```python
from build123d import *

# Parameters (mm, degrees)
SKETCH1_R           = 13.5
BOSS_EXTRUDE1_DEPTH = 3.25
CUT_EXTRUDE1_DEPTH  = 4.25
FILLET1_R           = 0.57
CIRPATTERN3_COUNT   = 16


with BuildPart() as part:
    # Sketch1 → Boss-Extrude1 (new body, symmetric)
    with BuildSketch(Plane.XY):
        Circle(SKETCH1_R)
        with BuildLine():
            Line((1.4, 1), (2.1, 1))
            ThreePointArc((2.1, 1), (2.382842712, 0.882842712), (2.5, 0.6))
            Line((2.5, 0.6), (2.5, -0.6))
            ThreePointArc((2.5, -0.6), (2.382842712, -0.882842712), (2.1, -1))
            Line((2.1, -1), (1.4, -1))
            ThreePointArc((1.4, -1), (1.117157288, -1.117157288), (1, -1.4))
            Line((1, -1.4), (1, -2.1))
            ThreePointArc((1, -2.1), (0.882842712, -2.382842712), (0.6, -2.5))
            Line((0.6, -2.5), (-0.6, -2.5))
            ThreePointArc((-0.6, -2.5), (-0.882842712, -2.382842712), (-1, -2.1))
            Line((-1, -2.1), (-1, -1.4))
            ThreePointArc((-1, -1.4), (-1.117157288, -1.117157288), (-1.4, -1))
            Line((-1.4, -1), (-2.1, -1))
            ThreePointArc((-2.1, -1), (-2.382842712, -0.882842712), (-2.5, -0.6))
            Line((-2.5, -0.6), (-2.5, 0.6))
            ThreePointArc((-2.5, 0.6), (-2.382842712, 0.882842712), (-2.1, 1))
            Line((-2.1, 1), (-1.4, 1))
            ThreePointArc((-1.4, 1), (-1.117157288, 1.117157288), (-1, 1.4))
            Line((-1, 1.4), (-1, 2.1))
            ThreePointArc((-1, 2.1), (-0.882842712, 2.382842712), (-0.6, 2.5))
            Line((-0.6, 2.5), (0.6, 2.5))
            ThreePointArc((0.6, 2.5), (0.882842712, 2.382842712), (1, 2.1))
            Line((1, 2.1), (1, 1.4))
            ThreePointArc((1, 1.4), (1.117157288, 1.117157288), (1.4, 1))
        make_face(mode=Mode.SUBTRACT)
    extrude(amount=BOSS_EXTRUDE1_DEPTH, both=True)

    # Sketch2 → Cut-Extrude1 (cut, symmetric)
    with BuildSketch(Plane.XY):
        with BuildLine():
            ThreePointArc((0.982234387, 10.077243701), (0, 10.125), (-0.982234387, 10.077243701))
            ThreePointArc((-0.982234387, 10.077243701), (-1.348268622, 11.771504161), (-2.092826994, 13.336794037))
            ThreePointArc((-2.092826994, 13.336794037), (0, 13.5), (2.092826994, 13.336794037))
            ThreePointArc((2.092826994, 13.336794037), (1.348268622, 11.771504161), (0.982234387, 10.077243701))
        make_face()
    cut_extrude1 = extrude(amount=CUT_EXTRUDE1_DEPTH, both=True, mode=Mode.SUBTRACT)

    # Fillet1
    fillet1_edges = [part.edges().sort_by_distance(p)[0] for p in [
        (-0.982234387, 10.077243701, 0),
        (0.982234387, 10.077243701, 0),
    ]]
    fillet(fillet1_edges, radius=FILLET1_R)

    # CirPattern3: Cut-Extrude1 ×16 about axis
    cirpattern3_axis = Axis((0, 0, 0), (0, 0, 1))
    for i in range(1, CIRPATTERN3_COUNT):
        add(cut_extrude1.rotate(cirpattern3_axis, i * 360 / CIRPATTERN3_COUNT), mode=Mode.SUBTRACT)


solid = part.part
```
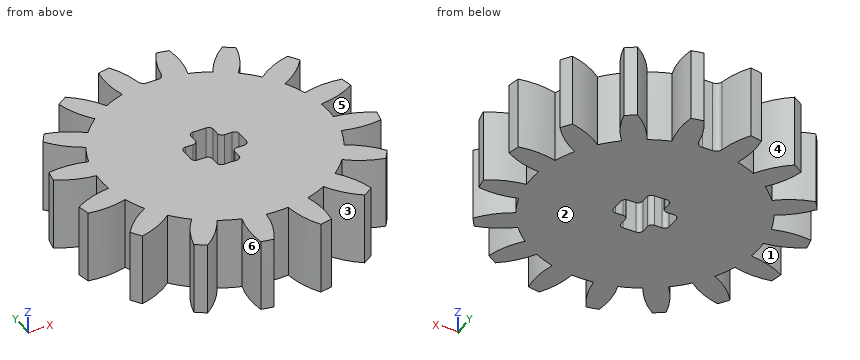
Design review of the part built by this model. Coordinates are the model's own, in mm. Face numbers are marked on the shaded views. A direction names the side the tool comes from. Give positions to 0.01 mm unless a question says otherwise; leave off trailing zeros. Order: outer loops, then holes, each group sorted by start corner. A loop starts at its lowest first (then second) coordinate and runs counter-clockwise, first axis right, second up. Notation, with made-up numbers: (-14.5, 54.5) - (19.5, 54.5) arc R11 ccw to (19.5, 72.5) - close; hole circle Ø2 at (78, 23.5). An arc over 180 degrees is marked (long way). Use a Markdown table: item, result. Add a question column.
(1) Add section A-A on y = 1.75. Give the boundary of the cut face in (x, z), then the cut area to 3 significant figures.
(2) Clearance check with flat-ended pins moving along their axes: P1, Ø1.3, axis at x = 0, z = -1, coming from the +Y side; P2, Ø0.8, axis at y = 2, z = 0, coming from the -X side; P3, Ø0.6, axis at y = 0, z = 0, coming from the +X side (3 decimals); P4, Ø0.8, axis at x = -1.5, z = -1.5, coming from the +Y side. State where each tip first meets the part, or that it passes through.
(3) Mouldability with a two-part tool opening along Y and no side actions: class the marked faces 1, 2 and 3 as +Y half, -Y half, draft (parallel to the pull), parting line (faces both ways), or undercut.
(4) Wall thickness on probe 1 along X at (y, z) = (-0.25, 1.25); probe 2 along X at (y, z) = (-11.25, 2.5); probe 3 along Y at (x, z) = (-11, -0.25): over which ranges is each line inside the solid? List them lowest first. Write a range as [from, to].
(5) Machinability: for the marked faces 4, 5 and 6, which of the approach directions +Z, -Z, +X, -X, +Y, -Y give a long, thin tool a straight path to every point of the face, cutting with its end or side? Answer none if there is none.
(6) Add section B-B on x = -8.5. Give the boundary of the cut face in (y, z).
Report:
| question | item | result |
|---|---|---|
| 1 | outline | (-12.73, -3.25) - (-1, -3.25) - (-1, 3.25) - (-12.73, 3.25) - close; (1, -3.25) - (12.73, -3.25) - (12.73, 3.25) - (1, 3.25) - close |
| 1 | area | 152 mm² |
| 2 | P1 | stops at y = 10.14 |
| 2 | P2 | stops at x = -13.34 |
| 2 | P3 | stops at x = 10.125 |
| 2 | P4 | stops at y = 13.01 |
| 3 | face 1 | undercut |
| 3 | face 2 | draft |
| 3 | face 3 | -Y half |
| 4 | probe 1 | x = [-10.12, -2.5], [2.5, 10.12] |
| 4 | probe 2 | x = [-7.46, -6.68], [-3.25, -1.19], [1.19, 3.25], [6.68, 7.46] |
| 4 | probe 3 | y = [-7.83, -6.39], [-3.22, -1.13], [1.13, 3.22], [6.39, 7.83] |
| 5 | face 4 | +Z, -Z, +Y |
| 5 | face 5 | +Z, -Z, +X |
| 5 | face 6 | +Z, -Z |
| 6 | outline | (-6.93, -3.25) - (6.93, -3.25) - (6.93, 3.25) - (-6.93, 3.25) - close |
